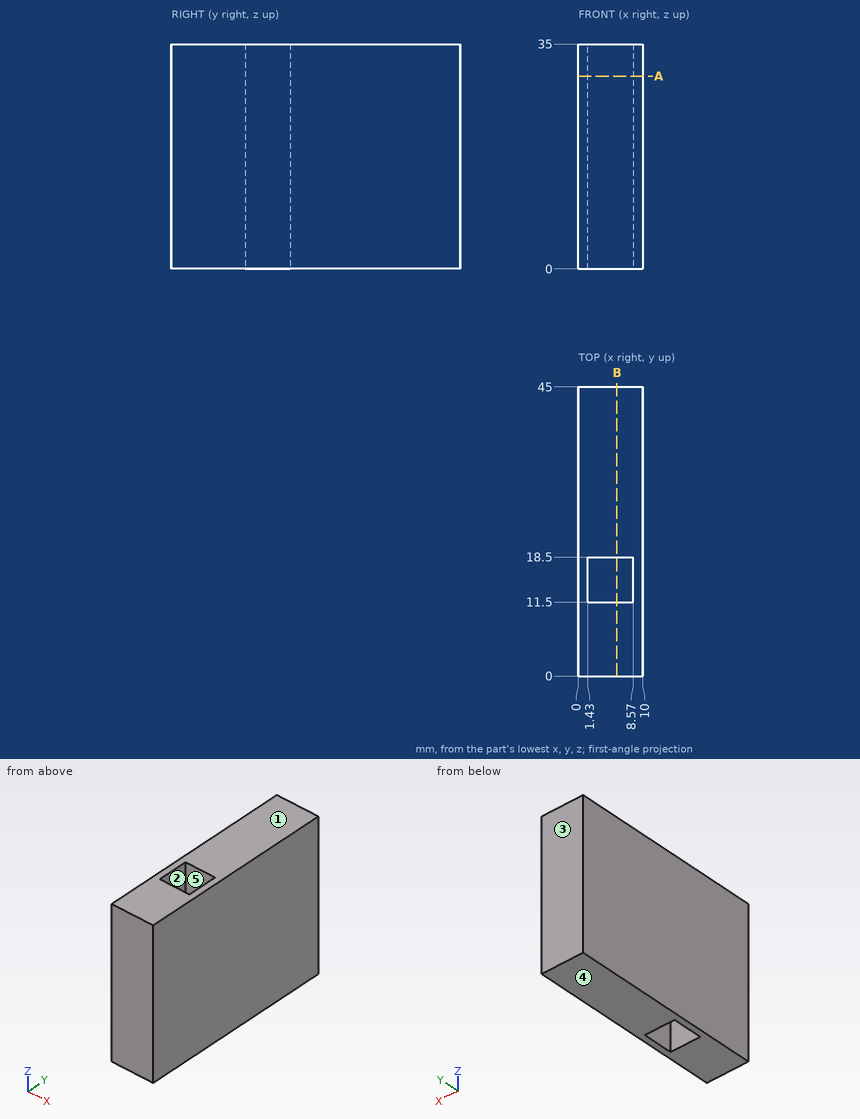
The figure shows three views and two pictorial views of one solid part (mm, origin at its lowest corner). Answer the questions. A direction names the side the tool comes from. Give positions to 0.01 mm unless a question says otherwise; leave off trailing zeros. Write each loop counter-clockwise with the first axis right and the second up, starting at its lowest first coordinate (ties: lowest second). Pieces come first, ordered by that corner, then holes. Notation, with made-up numbers: (-6, 74.5) -> (45, 74.5) arc R36 ccw to (45, 111.5) -> close; hole circle Ø3 at (34.25, -1.75). An arc over 180 degrees is marked (long way). Answer as a JSON object with one key per item and string values.
1) Section A-A on z = 30 is taken. Write down the section's boundary in (x, y), then the cut area to 3 significant figures.
Findings below:
{"outline": "(0, 0) -> (10, 0) -> (10, 45) -> (0, 45) -> close; hole (1.43, 11.5) -> (8.57, 11.5) -> (8.57, 18.5) -> (1.43, 18.5) -> close", "area": "400 mm^2"}
2) For a pull along Y with two mould halves and no side action, classify the marked faces 3, 4 and 5 as pulls with the +Y half, pulls with the -Y half, needs draft (parallel to the pull), parting line crosses it, or undercut.
Findings below:
{"face 3": "pulls with the +Y half", "face 4": "needs draft", "face 5": "undercut"}
3) Section B-B on x = 6 is taken. Write down the section's boundary in (y, z).
Findings below:
{"outline": "(0, 0) -> (11.5, 0) -> (11.5, 35) -> (0, 35) -> close; (18.5, 0) -> (45, 0) -> (45, 35) -> (18.5, 35) -> close"}
4) Straight lines are drawn through the part: probe 1 along X at (y, z) = (15.5, 27); probe 2 along Y at (x, z) = (8, 8.5). For each, find the intervals that lie inside material, in ascending order. Write a range as from..to.
Findings below:
{"probe 1": "x = 0..1.43, 8.57..10", "probe 2": "y = 0..11.5, 18.5..45"}
5) A tool of negligible diameter and unlimited length cuts with its end or side. For the marked faces 1 and 2, from which of +Z, -Z, +X, -X, +Y, -Y can it reach the whole face along a straight path? Write none if from no direction.
Findings below:
{"face 1": "+Z, +X, -X, +Y, -Y", "face 2": "+Z, -Z"}
